Input: part model. Units: mm. Frame: model coordinates. Face numbers are marked on the shaded views. A direction names the side the tool comes from. Coordinates: 2 decimals unless noted, no trailing zeros. Order: outer loops, then holes, each group sorted by start corner. A loop starts at its lowest first (then second) coordinate and runs counter-clockwise, first axis right, second up. Notation, with made-up numbers: (-15, 44) -> (38, 44) arc R18 ccw to (38, 61) -> close; hole circle Ø3 at (64, 34). An arc over 180 degrees is marked (long way). One line per item, written item: value. Start each with the question number.
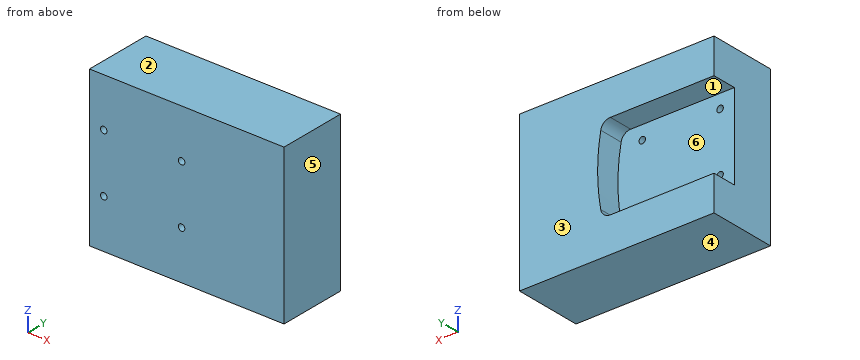
from build123d import *

# Parameters (mm, degrees)
SKETCH1_W           = 127
SKETCH1_H           = 101.6
BOSS_EXTRUDE1_DEPTH = 44.45
CUT_EXTRUDE1_DEPTH  = 16
SKETCH3_R           = 2.1082
CUT_EXTRUDE2_DEPTH  = 87.152727757


with BuildPart() as part:
    # Sketch1 → Boss-Extrude1 (new body)
    with BuildSketch(Plane(origin=(0, 0, 0), x_dir=(1, 0, 0), z_dir=(0, 1, 0))):
        Rectangle(SKETCH1_W, SKETCH1_H)
    extrude(amount=BOSS_EXTRUDE1_DEPTH)

    # Sketch2 → Cut-Extrude1 (cut)
    with BuildSketch(Plane(origin=(0, 44.45, 0), x_dir=(1, 0, 0), z_dir=(0, 1, 0))):
        with BuildLine():
            Line((-63.5, 28), (4.191617227, 28))
            ThreePointArc((4.191617227, 28), (8.25897768, 26.526379697), (10.43854445, 22.789473684))
            ThreePointArc((10.43854445, 22.789473684), (12.5, 0), (10.43854445, -22.789473684))
            ThreePointArc((10.43854445, -22.789473684), (8.25897768, -26.526379697), (4.191617227, -28))
            Line((4.191617227, -28), (-63.5, -28))
            Line((-63.5, -28), (-63.5, 28))
        make_face()
    extrude(amount=-CUT_EXTRUDE1_DEPTH, mode=Mode.SUBTRACT)

    # Sketch3 → Cut-Extrude2 (cut, through all)
    with BuildSketch(Plane(origin=(0, 28.45, 0), x_dir=(1, 0, 0), z_dir=(0, 1, 0))):
        with Locations(Location((-54.175, 19.05, 0), (0, 0, 270))):
            Circle(SKETCH3_R)
        with Locations(Location((-54.175, -19.05, 0), (0, 0, 270))):
            Circle(SKETCH3_R)
        with Locations(Location((-3.375, 19.05, 0), (0, 0, 270))):
            Circle(SKETCH3_R)
        with Locations(Location((-3.375, -19.05, 0), (0, 0, 270))):
            Circle(SKETCH3_R)
    extrude(amount=-CUT_EXTRUDE2_DEPTH, mode=Mode.SUBTRACT)


solid = part.part
1) Pin query (flat end, axial travel): pin 1 Ø3.5 at (x, z) = (-3.375, 19.05) entering from -Y; pin 2 Ø10 at (x, z) = (-38.5, 16) entering from +Y. Return the tip coordinate at first contact, or that it passes through.
2) Ray query, line 1 along X through (y, z) = (14.5, -19.05); line 2 along Z through (x, y) = (-17.5, 38.5); line 3 along Y through (x, z) = (-37, 11.5). Return the intervals inside material, ascending. Write a range as from..to.
3) Section query B-B, the plane y = 41. Return the cut outline in (x, z), plus the area to 3 significant figures.
4) Mould query, pull axis Z, two halves, no side actions, for the marked faces 1, 2, 3 and 4. Classes: +Z half, -Z half, draft (parallel to the pull), parting line (faces both ways), or undercut.
5) Section query C-C, the plane z = 6. Return the cut outline in (x, y).
6) Access query for the marked faces 5 and 6. Directions: +Z, -Z, +X, -X, +Y, -Y. A direction counts if a zero-diameter tool reaches every point of the face in a straight line with its end or side. Return the directions, or none.
7) Section query A-A, the plane z = 19.05. Return the cut outline in (x, y), plus the area to 3 significant figures.
Entries:
1. pin 1: passes through
1. pin 2: stops at y = 28.45
2. line 1: x = -63.5..-56.28, -52.07..-5.48, -1.27..63.5
2. line 2: z = -50.8..-28, 28..50.8
2. line 3: y = 0..28.45
3. outline: (-63.5, -50.8) -> (63.5, -50.8) -> (63.5, 50.8) -> (-63.5, 50.8) -> (-63.5, 28) -> (4.19, 28) arc R6.35 cw to (10.44, 22.79) arc R127 cw to (10.44, -22.79) arc R6.35 cw to (4.19, -28) -> (-63.5, -28) -> close
3. area: 8,720 mm2
4. face 1: undercut
4. face 2: +Z half
4. face 3: draft
4. face 4: -Z half
5. outline: (-63.5, 0) -> (63.5, 0) -> (63.5, 44.45) -> (12.36, 44.45) -> (12.36, 28.45) -> (-63.5, 28.45) -> close
6. face 5: +Z, -Z, +X, +Y, -Y
6. face 6: -X, +Y
7. outline: (-63.5, 0) -> (-56.28, 0) -> (-56.28, 28.45) -> (-63.5, 28.45) -> close; (-52.07, 0) -> (-5.48, 0) -> (-5.48, 28.45) -> (-52.07, 28.45) -> close; (-1.27, 0) -> (63.5, 0) -> (63.5, 44.45) -> (11.06, 44.45) -> (11.06, 28.45) -> (-1.27, 28.45) -> close
7. area: 4,210 mm2
